Work out the finished part from the listing and answer in its coordinate system (mm). A direction names the side the tool comes from. Coordinates: 2 decimals unless noted, no trailing zeros. Order: outer loops, then holes, each group sorted by start corner. A loop starts at its lowest first (then second) coordinate and runs counter-clockwise, first axis right, second up. Notation, with made-up numbers: (-28, -21.5) - (23, -21.5) arc R34 cw to (23, 13.5) - close; hole circle Ø5 at (75, -5). An arc over 180 degrees is marked (long way). Answer as a JSON object with one key per item and string values. Group by question number.
1) Section B-B (z = 29) is taken. Give the vertices of the cut face in (x, y) (1 decimal), plus the area to 3 significant figures.
2) A tool of negligible diameter and unlimited length cuts with its end or side. For faces 1 (the face through (17.19, -1.388, 39.165)), 2 (the face through (-18, -0.4, 19.2)), 3 (the face through (19.96, -0.64, 40.96)), 4 (the face through (-25.31, -4.71, 44.15)), 5 (the face through (0.806, -8.476, 6.179)), from which of +Z, -Z, +X, -X, +Y, -Y can it reach the whole face along a straight path? Write none if from no direction.
3) Each of these flat-tipped pins is pushed along its axis until it touches: P1, Ø2, axis at x = -20.5, y = -1, coming from the -Z side (3 decimals); P2, Ø1.9, axis at x = 17.5, z = 38.5, coming from the -Y side; P3, Ø2, axis at x = -20.5, y = -1, coming from the +Z side; P4, Ø7, axis at x = 18.5, z = 40.5, coming from the +Y side. Where does it stop, or does it pass through?
4) Section A-A (x = -13) is taken. Give the vertices of the cut face in (y, z) (3 decimals), plus the area to 3 significant figures.
5) The mould has two halves that part along X. Classify faces 6 (the face through (22.9, -0.39, 27.71)), 7 (the face through (-19.947, -4.456, 40.738)), 8 (the face through (-18.3, -4.7, 19)): released by +X, released by -X, zero draft, split by the parting line, or undercut.
6) Find the intervals of material crossed by line 1 along Z through (x, y) = (-1.5, -7.25); line 2 along X through (y, z) = (-8, 34.5); line 3 along X through (y, z) = (-2, 31), in increasing order.
from build123d import *

# Parameters (mm, degrees)
F1_DEPTH     = 9.525
F3_T1_DEPTH  = 28.8029547439
F3_T3_DEPTH  = 22.5439921386
F3_T5_DEPTH  = 28.8029547439
F3_T8_ANGLE  = 120
F3_T10_ANGLE = 120
F3_T12_ANGLE = 149.490366343
F5_DEPTH     = 9.525
F6_SIZE      = 0.762
F8_R         = 3.175
F9_DEPTH     = 9.526
F10_SIZE     = 0.762
F12_DEPTH    = 1.27


# Not quite as in the source:
# - a fillet or chamfer that OpenCascade refuses, or shapes differently, is made with other operations: its cross-section is extruded or revolved along the edge and cut away or added
# - a feature of the source that left no trace in its solid (it failed there, or was rolled back) is left out
# - a feature names something its author has since deleted; it is built from what else it names


with BuildPart() as f1:
    # F0 (on Front) → F1 (new body)
    with BuildSketch(Plane.XZ):
        with BuildLine():
            Line((-14.4014773719, 43.9940905122), (14.4014773719, 43.9940905122))
            ThreePointArc((14.4014773719, 43.9940905122), (19.900738686, 40.8190905122), (19.900738686, 34.4690905122))
            Line((19.900738686, 34.4690905122), (10.261761314, 17.773891971))
            ThreePointArc((10.261761314, 17.773891971), (11.423891971, 13.436761314), (15.7610226281, 14.598891971))
            Line((15.7610226281, 14.598891971), (25.4, 31.2940905122))
            ThreePointArc((25.4, 31.2940905122), (25.4, 43.9940905122), (14.4014773719, 50.3440905122))
            Line((14.4014773719, 50.3440905122), (-14.4014773719, 50.3440905122))
            ThreePointArc((-14.4014773719, 50.3440905122), (-25.4, 43.9940905122), (-25.4, 31.2940905122))
            Line((-25.4, 31.2940905122), (-10.9985226281, 6.35))
            ThreePointArc((-10.9985226281, 6.35), (0, 0), (10.9985226281, 6.35))
            ThreePointArc((10.9985226281, 6.35), (9.836391971, 10.687130657), (5.499261314, 9.525))
            ThreePointArc((5.499261314, 9.525), (0, 6.35), (-5.499261314, 9.525))
            Line((-5.499261314, 9.525), (-19.900738686, 34.4690905122))
            ThreePointArc((-19.900738686, 34.4690905122), (-19.900738686, 40.8190905122), (-14.4014773719, 43.9940905122))
        make_face()
    extrude(amount=F1_DEPTH)

    # F3: chamfer of 1.27 on 6 edges, made by hand

    # F3_s2 → F3_t1 (cut)
    with BuildSketch(Plane.YZ.offset(-14.4014773719)):
        Polygon((-8.255, 43.9940905122), (-9.525, 45.2640905122), (-9.525, 43.9940905122), align=None)
    extrude(amount=F3_T1_DEPTH, mode=Mode.SUBTRACT)

    # F3_s4 → F3_t3 (cut)
    with BuildSketch(Plane(origin=(19.900738686, 0, 34.4690905122), x_dir=(0, 1, 0), z_dir=(-0.5, 0, -0.8660254038))):
        Polygon((-8.255, 0), (-9.525, 1.27), (-9.525, 0), align=None)
    extrude(amount=F3_T3_DEPTH, mode=Mode.SUBTRACT)

    # F3_s6 → F3_t5 (cut)
    with BuildSketch(Plane(origin=(-5.499261314, 0, 9.525), x_dir=(0, 1, 0), z_dir=(-0.5, 0, 0.8660254038))):
        Polygon((-8.255, 0), (-9.525, 1.27), (-9.525, 0), align=None)
    extrude(amount=F3_T5_DEPTH, mode=Mode.SUBTRACT)

    # F3_s7 → F3_t8 (revolve, cut)
    with BuildSketch(Plane(origin=(-19.900738686, 0, 34.4690905122), x_dir=(0, 1, 0), z_dir=(0.5, 0, -0.8660254038))):
        Polygon((-8.255, 0), (-9.525, -1.27), (-9.525, 0), align=None)
    revolve(axis=Axis((-14.4014773719, -9.525, 37.6440905122), (0, 1, 0)), revolution_arc=F3_T8_ANGLE, mode=Mode.SUBTRACT)

    # F3_s9 → F3_t10 (revolve, cut)
    with BuildSketch(Plane.YZ.offset(14.4014773719)):
        Polygon((-8.255, 43.9940905122), (-9.525, 45.2640905122), (-9.525, 43.9940905122), align=None)
    revolve(axis=Axis((14.4014773719, -9.525, 37.6440905122), (0, 1, 0)), revolution_arc=F3_T10_ANGLE, mode=Mode.SUBTRACT)

    # F3_s11 → F3_t12 (revolve, cut)
    with BuildSketch(Plane(origin=(0.1129578151, 0, 12.698995238), x_dir=(0, 1, 0), z_dir=(0.008894668, 0, 0.9999604417))):
        Polygon((-8.255, -6.2370377163), (-9.525, -7.5070377163), (-9.525, -6.2370377163), align=None)
    revolve(axis=Axis((0, -9.525, 12.7), (0, 1, 0)), revolution_arc=F3_T12_ANGLE, mode=Mode.SUBTRACT)

    # F4 (on face) → F5 (join, through all)
    with BuildSketch(Plane(origin=(0, 0, 0), x_dir=(-1, 0, 0), z_dir=(0, 1, 0))):
        with BuildLine():
            Line((-30.899261314, 40.8190905122), (-25.4, 31.2940905122))
            ThreePointArc((-25.4, 31.2940905122), (-25.4, 43.9940905122), (-14.4014773719, 50.3440905122))
            Line((-14.4014773719, 50.3440905122), (-25.4, 50.3440905122))
            ThreePointArc((-25.4, 50.3440905122), (-30.899261314, 47.1690905122), (-30.899261314, 40.8190905122))
        make_face()
    extrude(amount=-F5_DEPTH)

    # F6
    f6_edges = [f1.edges().sort_by_distance(p)[0] for p in [
        (12.821161, -9.525, 13.017096),
        (23.330142, -9.525, 27.708991),
        (30.899261, -9.525, 47.169091),
        (5.499261, -9.525, 50.344091),
        (-25.4, -9.525, 43.994091),
        (-18.199261, -9.525, 18.822045),
        (0, -9.525, 0),
        (10.76839, -9.525, 9.869534),
        (9.836392, 0, 10.687131),
        (0, 0, 0),
        (-18.199261, 0, 18.822045),
        (-25.4, 0, 43.994091),
        (5.499261, 0, 50.344091),
        (30.899261, 0, 47.169091),
        (23.330142, 0, 27.708991),
        (11.423892, 0, 13.436761),
        (15.08125, 0, 26.121491),
        (19.900739, 0, 40.819091),
        (0, 0, 43.994091),
        (-19.900739, 0, 40.819091),
        (-12.7, 0, 21.997045),
        (0, 0, 6.35),
    ]]
    chamfer(f6_edges, length=F6_SIZE)

    # F8 (on face) → F9 (cut, through all)
    with BuildSketch(Plane.XZ.offset(9.525)):
        with Locations((25.6199704526, 44.1210905122)):
            Circle(F8_R)
    extrude(amount=-F9_DEPTH, mode=Mode.SUBTRACT)

    # F10
    f10_edges = [f1.edges().sort_by_distance(p)[0] for p in [
        (22.44497, -9.525, 44.121091),
        (28.79497, -4.7625, 44.121091),
        (22.44497, 0, 44.121091),
    ]]
    chamfer(f10_edges, length=F10_SIZE)

    # F11 (on offset) → F12 (join)
    with BuildSketch(Plane(origin=(0, -0.762, 0), x_dir=(-1, 0, 0), z_dir=(0, 1, 0))):
        with BuildLine():
            Line((-19.900738686, 34.4690905122), (-14.4014773719, 43.9940905122))
            ThreePointArc((-14.4014773719, 43.9940905122), (-19.900738686, 40.8190905122), (-19.900738686, 34.4690905122))
        make_face()
    extrude(amount=-F12_DEPTH)


solid = f1.part
Report:
{
 "1": {"outline": "(-24.1, -8.8) - (-23.2, -9.5) - (-18.2, -9.5) - (-16.7, -8.3) - (-16.7, -0.8) - (-17.6, 0) - (-23.2, 0) - (-24.1, -0.8) - close; (16.7, -8.3) - (18.2, -9.5) - (23.2, -9.5) - (24.1, -8.8) - (24.1, -0.8) - (23.2, 0) - (17.6, 0) - (16.7, -0.8) - close", "area": "136 mm²"},
 "2": {"face 1": "+Y, -Y", "face 2": "-Z, -X, +Y", "face 3": "+Y", "face 4": "-X, +Y, -Y", "face 5": "-Y"},
 "3": {"P1": "stops at z = 21.075", "P2": "stops at y = -2.03", "P3": "stops at z = 49.28", "P4": "stops at y = 0"},
 "4": {"outline": "(-9.525, 11.341) - (-8.763, 9.817) - (-0.762, 9.817) - (0, 11.341) - (0, 20.993) - (-0.762, 22.517) - (-8.255, 22.517) - (-9.525, 19.977) - close; (-9.525, 45.264) - (-8.255, 43.994) - (-0.762, 43.994) - (0, 44.756) - (0, 49.582) - (-0.762, 50.344) - (-8.763, 50.344) - (-9.525, 49.582) - close", "area": "176 mm²"},
 "5": {"face 6": "released by +X", "face 7": "undercut", "face 8": "released by -X"},
 "6": {"line 1": "z = 0.09 to 6.53, 43.99 to 50.34", "line 2": "x = -26.71 to -19.92, 19.92 to 27.25", "line 3": "x = -25.23 to -17.9, 17.9 to 25.23"}
}
